```python
from build123d import *

# Parameters (mm, degrees)
F0_R          = 500
F1_DEPTH      = 914
F1_DEPTH_BACK = 914
F2_R          = 100
F4_W          = 100
F4_H          = 150
F5_DEPTH      = 283.055052823
F5_DEPTH_BACK = 50
F7_R          = 19.05
F8_DEPTH      = 25


with BuildPart() as f1:
    # F0 (on Front) → F1 (new body, two sides)
    with BuildSketch(Plane.XZ) as f1_sk:
        Circle(F0_R)
    extrude(amount=F1_DEPTH)
    extrude(f1_sk.sketch, amount=-F1_DEPTH_BACK)

    # F2
    f2_edges = [f1.edges().sort_by_distance(p)[0] for p in [
        (-500, -914, 0),
        (-500, 914, 0),
    ]]
    fillet(f2_edges, radius=F2_R)

    # F4 (on offset) → F5 (join, two sides)
    with BuildSketch(Plane.XY.offset(500)) as f5_sk:
        with Locations((-400, 575)):
            Rectangle(F4_W, F4_H)
        with Locations((400, 575)):
            Rectangle(F4_W, F4_H)
        with Locations((400, -575)):
            Rectangle(F4_W, F4_H)
        with Locations((-400, -575)):
            Rectangle(F4_W, F4_H)
    extrude(amount=-F5_DEPTH)
    extrude(f5_sk.sketch, amount=F5_DEPTH_BACK)

    # F7 (on offset) → F8 (cut)
    with BuildSketch(Plane.XY.offset(-500)):
        with Locations((0, -600)):
            Circle(F7_R)
        with Locations((0, -500)):
            Circle(F7_R)
        with Locations((0, -400)):
            Circle(F7_R)
        with Locations((0, 500)):
            Circle(F7_R)
        with Locations((0, 400)):
            Circle(F7_R)
        with Locations((0, 600)):
            Circle(F7_R)
    extrude(amount=F8_DEPTH, mode=Mode.SUBTRACT)


solid = f1.part
```
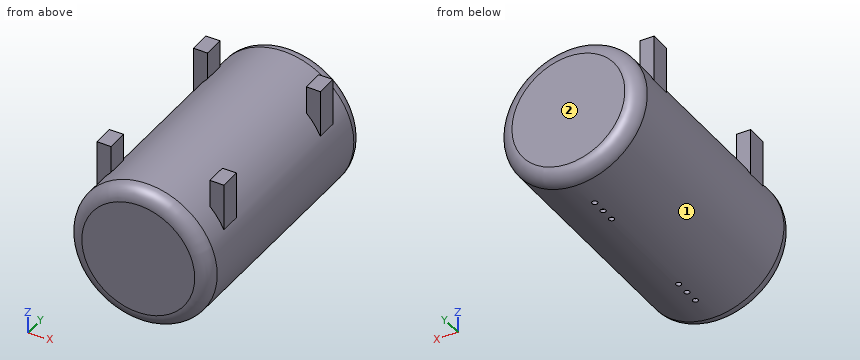
Input: part model. Units: mm. Frame: model coordinates. Face numbers are marked on the shaded views. Coordinates: 2 decimals unless noted, no trailing zeros. Loops run counter-clockwise (first coordinate to the right, second up) from the corner with the lowest first, then second, coordinate; pieces in that order, holes last. Notation, with made-up numbers: (-20.5, 36) -> (22.5, 36) arc R23 ccw to (22.5, 63) -> close; hole circle Ø6 at (-38.75, -7.5). An arc over 180 degrees is marked (long way). Use a Markdown table: item, result.
1) Cut plane A-A (y = -210.5). Return the cut outline in (x, z), then the cut area to 3 significant figures.
Results found:
| item | result |
|---|---|
| outline | circle Ø1000 at (0, 0) |
| area | 785,000 mm2 |
2) Contact query for flat-ended pins moving along their axis: pin 1 (12 mm diameter, centred on x = -369.5, z = 393, fed in from +Y); pin 2 (4 mm diameter, centred on x = 347.5, y = -30, fed in from +Z); pin 3 (2 mm diameter, centred on x = 205.5, y = -506, fed in from -Z). Output: stop coordinate, or through.
Results found:
| item | result |
|---|---|
| pin 1 | stops at y = 650 |
| pin 2 | stops at z = 361.43 |
| pin 3 | stops at z = -456.27 |
3) Cut plane B-B (y = -600). Return the cut outline in (x, z), then the cut area to 3 significant figures.
Results found:
| item | result |
|---|---|
| outline | (-450, 217.94) arc R500 ccw to (-19.05, -499.64) -> (-19.05, -475) -> (19.05, -475) -> (19.05, -499.64) arc R500 ccw to (450, 217.94) -> (450, 550) -> (350, 550) -> (350, 357.07) arc R500 ccw to (-350, 357.07) -> (-350, 550) -> (-450, 550) -> close |
| area | 835,000 mm2 |
4) Material intervals for line 1 along Y through (x, z) = (357, 353); line 2 along Z through (x, y) = (-12, -51); line 3 along X through (y, z) = (619, 282), sorted ascending. Write a range as from..to.
Results found:
| item | result |
|---|---|
| line 1 | y = -650..-500, 500..650 |
| line 2 | z = -499.86..499.86 |
| line 3 | x = -450..450 |
5) Pull-direction query (Z, two-part tool) for the marked faces 1 and 2; classes: released by +Z, released by -Z, zero draft, split by the parting line, or undercut.
Results found:
| item | result |
|---|---|
| face 1 | split by the parting line |
| face 2 | zero draft |
6) Cut plane C-C (y = -400). Return the cut outline in (x, z), then the cut area to 3 significant figures.
Results found:
| item | result |
|---|---|
| outline | (-19.05, -499.64) -> (-19.05, -475) -> (19.05, -475) -> (19.05, -499.64) arc R500 ccw (long way) to start |
| area | 784,000 mm2 |
